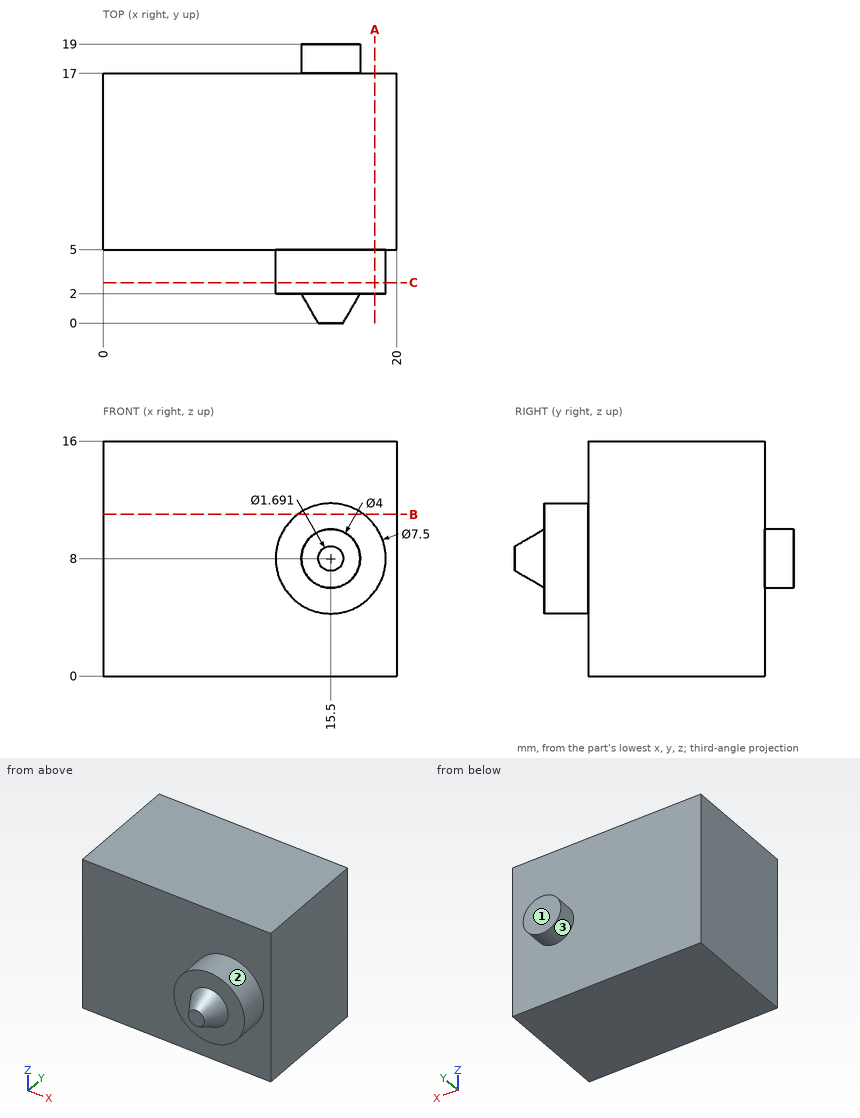
Could you check a few things on this drawing? It's one solid part, dimensions in mm from its lowest x, y, z. A direction names the side the tool comes from. Round coordinates to 2 decimals unless told otherwise and drop trailing zeros. Loops run counter-clockwise (first coordinate to the right, second up) from the corner with the lowest first, then second, coordinate; pieces in that order, holes last.
Q1. I want a section at B-B (z = 11). Write out the boundary of the cut face in (x, y).
Q2. Please list where these lines run through material, in increasing order: L1, parallel to Y at x = 11.25, z = 11.25; L2, parallel to Y at x = 12, z = 7.5; L3, parallel to X at y = 3.75, z = 5.
Q3. For P1, Ø5, axis at x = 8.5, z = 5, coming from the +Y side; P2, Ø2, axis at x = 7.5, z = 12, coming from the -Y side; P3, Ø1.5, axis at x = 13.5, y = 2.5, coming from the +Z side (1 decimal), each with a flat end and sliding along its axis, tell me the tip position at first contact or that it passes through.
Q4. I want a section at A-A (x = 18.5). Write out the boundary of the cut face in (y, z).
Q5. On a 3-axis mill with a long thin cutter (end or side, diameter ignored), from which of +Z, -Z, +X, -X, +Y, -Y can I reach the whole of each face in a straight line? I mean the marked faces 1, 2 and 3. Say none if no direction works.
Q6. I want a section at C-C (y = 2.75). Write out the boundary of the cut face in (x, z).
Answer below:
1. outline: (0, 5) - (13.25, 5) - (13.25, 2) - (17.75, 2) - (17.75, 5) - (20, 5) - (20, 17) - (0, 17) - close
2. L1: y = 5 to 17
2. L2: y = 2 to 17
2. L3: x = 13.25 to 17.75
3. P1: stops at y = 17
3. P2: stops at y = 5
3. P3: stops at z = 11.5
4. outline: (2, 5.75) - (5, 5.75) - (5, 0) - (17, 0) - (17, 16) - (5, 16) - (5, 10.25) - (2, 10.25) - close
5. face 1: +Z, -Z, +X, -X, +Y
5. face 2: -Y
5. face 3: +Y
6. outline: circle Ø7.5 at (15.5, 8)
